The figure shows three views and two pictorial views of one solid part (mm, origin at its lowest corner). Answer the questions. Coordinates: 2 decimals unless noted, no trailing zeros. Write each loop counter-clockwise with the first axis right and the second up, starting at its lowest first coordinate (ties: lowest second). Pieces come first, ordered by that corner, then holes.
Item 1: Straight lines are drawn through the part: probe 1 along Y at (x, z) = (10, 24.5); probe 2 along Z at (x, y) = (17.5, 12); probe 3 along X at (y, z) = (15.75, 8). For each, find the intervals that lie inside material, in ascending order.
Item 2: Section C-C (z = 32) is taken. Give the vertices of the cut face in (x, y).
Item 3: Determine the mould class of the marked faces 1, 2 and 3 for opening direction Y: released by +Y, released by -Y, zero draft, split by the parting line, or undercut.
Item 4: Each of these flat-tipped pins is pushed along its axis until it touches: P1, Ø1, axis at y = 2.5, z = 13, coming from the -X side; P2, Ø5, axis at y = 6, z = 24, coming from the +X side; P3, Ø4, axis at x = 9, y = 7, coming from the +Z side. Where does it stop, or does it pass through?
Item 5: Section A-A (y = 10) is taken. Give the vertices of the cut face in (x, z).
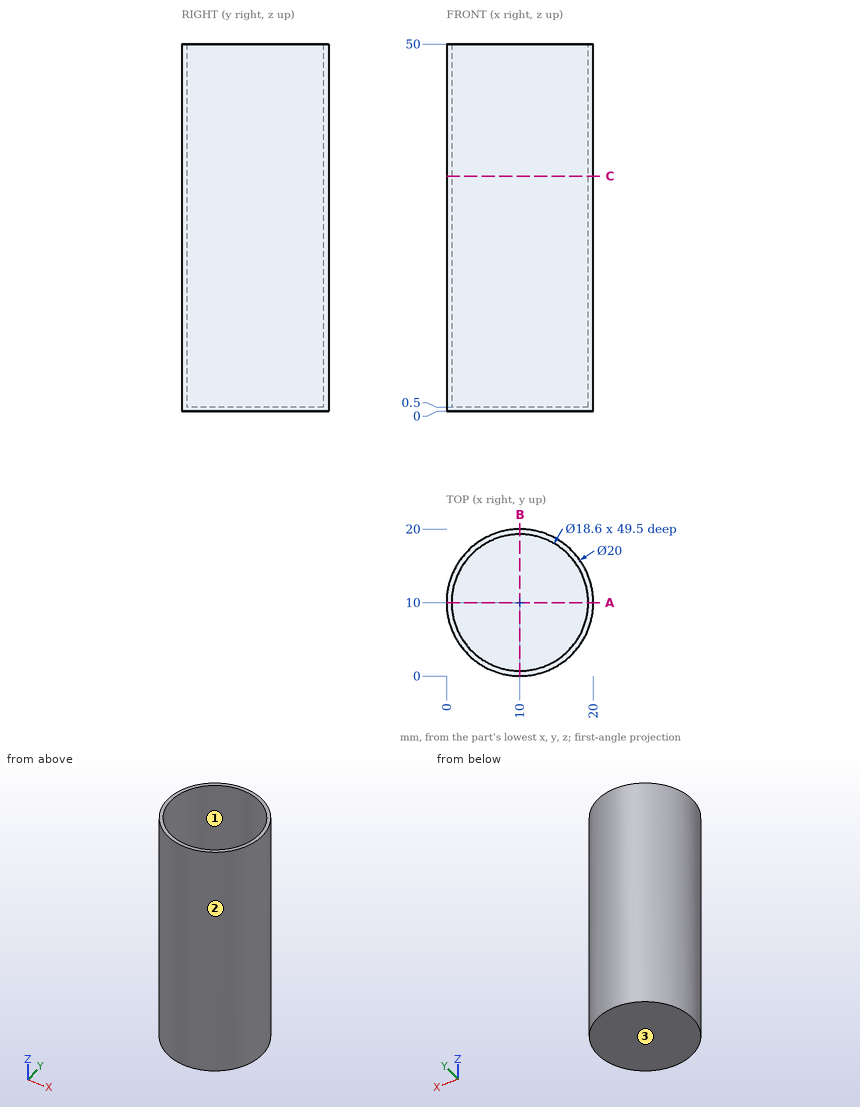
Established:
1. probe 1: y = 0 to 0.7, 19.3 to 20
1. probe 2: z = 0 to 0.5
1. probe 3: x = 1.82 to 2.69, 17.31 to 18.18
2. outline: circle Ø20 at (10, 10); hole circle Ø18.6 at (10, 10)
3. face 1: undercut
3. face 2: split by the parting line
3. face 3: zero draft
4. P1: stops at x = 2.86
4. P2: stops at x = 19.89
4. P3: stops at z = 0.5
5. outline: (0, 0) - (20, 0) - (20, 50) - (19.3, 50) - (19.3, 0.5) - (0.7, 0.5) - (0.7, 50) - (0, 50) - close
